from build123d import *

# Parameters (mm, degrees)
F0_W     = 30.48
F0_H     = 40.64
F1_DEPTH = 1.5748
F2_R     = 1.5875
F3_DEPTH = 1.5758
F4_W     = 19.8882
F4_H     = 27.686
F5_DEPTH = 8.382
F7_DEPTH = 0.635


with BuildPart() as f1:
    # F0 (on Front) → F1 (new body)
    with BuildSketch(Plane.XZ):
        Rectangle(F0_W, F0_H)
    extrude(amount=F1_DEPTH)

    # F2 (on face) → F3 (cut, through all)
    with BuildSketch(Plane.XZ.offset(1.5748)):
        with Locations((-12.065, 17.145)):
            Circle(F2_R)
        with Locations((12.065, 17.145)):
            Circle(F2_R)
        with Locations((-12.065, -17.145)):
            Circle(F2_R)
        with Locations((12.065, -17.145)):
            Circle(F2_R)
    extrude(amount=-F3_DEPTH, mode=Mode.SUBTRACT)

    # F4 (on face) → F5 (join)
    with BuildSketch(Plane.XZ.offset(1.5748)):
        Rectangle(F4_W, F4_H)
    extrude(amount=F5_DEPTH)

    # F6 (on face) → F7 (cut)
    with BuildSketch(Plane.XZ.offset(9.9568)):
        Polygon((-5.022132, -7.7724), (-5.250595, -9.398), (4.909405, -9.398), (7.737403, 10.724247), (-2.422597, 10.724247), (-3.708468, 1.5748), align=None)
        Polygon((-2.297791, -0.0508), (1.2573, -0.0508), (4.581493, -0.0508), (3.496293, -7.7724), (-3.382992, -7.7724), align=None, mode=Mode.SUBTRACT)
        Polygon((4.809956, 1.5748), (1.2573, 1.5748), (-2.069328, 1.5748), (-1.011921, 9.098647), (5.867364, 9.098647), align=None, mode=Mode.SUBTRACT)
        Polygon((-5.024567, -7.7724), (-5.022132, -7.7724), (-3.708468, 1.5748), (-3.710904, 1.5748), align=None)
    extrude(amount=-F7_DEPTH, mode=Mode.SUBTRACT)


solid = f1.part
Source: CAD feature listing. Evaluate the final solid. Frame: model axes, mm. A direction names the side the tool comes from. Round coordinates to 2 decimals unless told otherwise and drop trailing zeros. Loops run counter-clockwise (first coordinate to the right, second up) from the corner with the lowest first, then second, coordinate; pieces in that order, holes last. Notation, with made-up numbers: (-8.5, -11.5) - (-0.5, -11.5) arc R30 cw to (-0.5, 26.5) - close; hole circle Ø1 at (-21.5, 29.25). An arc over 180 degrees is marked (long way). Write item = value, one per line. Start each with the question number.
Item 1: Section query D-D on y = -6.5. Output: boundary loops of the cut face in (x, z), plus the area to 3 significant figures.
Item 2: Section query C-C on x = 0. Output: boundary loops of the cut face in (y, z).
Item 3: Section query B-B on x = 11.5. Output: boundary loops of the cut face in (y, z).
Item 4: Mould query, pull axis X, two halves, no side actions, for faces 4 (the face through (-15.24, -1, 0)), 5 (the face through (15.24, -1, 0)), 6 (the face through (-2.85, -9.64, -3.97)), 7 (the face through (0, 0, 0)). Classes: released by +X, released by -X, zero draft, split by the parting line, or undercut.
Item 5: Section query A-A on z = -12.5. Output: boundary loops of the cut face in (x, y).
Item 6: Reachability of faces 1 (the face through (6.3, -9.6, 0.5)), 2 (the face through (-10.599, -0.798, -17.753)), 3 (the face through (0, -6, 13.843)) from +Z, -Z, +X, -X, +Y, -Y: full face, straight path, thin tool, end or side. Return the list, or none.
Item 7: Material intervals for line 1 (X direction, y = -3, z = 10); line 2 (Z direction, x = 7, y = -3.5); line 3 (Y direction, x = -4, z = 17.5), sorted ascending.
Item 8: First-contact query: pin 1 Ø0.5 at (x, y) = (1.5, -9.5) entering from +Z; pin 2 Ø3.5 at (x, z) = (-12.065, -17.145) entering from -Y; pin 3 Ø1.9 at (x, z) = (12.065, 17.145) entering from -Y; pin 4 Ø1.5 at (x, y) = (8.5, -3) entering from -Z. Flat tips, straight axial feed; report the tip coordinate or a pass-through.
Results list:
q1.outline = (-9.94, -13.84) - (9.94, -13.84) - (9.94, 13.84) - (-9.94, 13.84) - close
q1.area = 551 mm²
q2.outline = (-9.96, -13.84) - (-1.57, -13.84) - (-1.57, -20.32) - (0, -20.32) - (0, 20.32) - (-1.57, 20.32) - (-1.57, 13.84) - (-9.96, 13.84) - (-9.96, 10.72) - (-9.32, 10.72) - (-9.32, 9.1) - (-9.96, 9.1) - (-9.96, 1.57) - (-9.32, 1.57) - (-9.32, -0.05) - (-9.96, -0.05) - (-9.96, -7.77) - (-9.32, -7.77) - (-9.32, -9.4) - (-9.96, -9.4) - close
q3.outline = (-1.57, -20.32) - (0, -20.32) - (0, -18.63) - (-1.57, -18.63) - close; (-1.57, -15.66) - (0, -15.66) - (0, 15.66) - (-1.57, 15.66) - close; (-1.57, 18.63) - (0, 18.63) - (0, 20.32) - (-1.57, 20.32) - close
q4.face_4 = released by -X
q4.face_5 = released by +X
q4.face_6 = undercut
q4.face_7 = zero draft
q5.outline = (-15.24, -1.57) - (-9.94, -1.57) - (-9.94, -9.96) - (9.94, -9.96) - (9.94, -1.57) - (15.24, -1.57) - (15.24, 0) - (-15.24, 0) - close
q6.face_1 = -Y
q6.face_2 = +Y, -Y
q6.face_3 = +Z, +X, -X, -Y
q7.line_1 = -9.94 to 9.94
q7.line_2 = -13.84 to 13.84
q7.line_3 = -1.57 to 0
q8.pin_1 = 13.84
q8.pin_2 = -1.57
q8.pin_3 = through
q8.pin_4 = -13.84
